```python
from build123d import *

# Parameters (mm, degrees)
BOSS_EXTRUDE1_DEPTH = 15
SKETCH3_R           = 5
CUT_EXTRUDE1_DEPTH  = 13
CUT_EXTRUDE2_START  = -7
SKETCH4_R           = 10.1
CUT_EXTRUDE2_DEPTH  = 2.6
SKETCH5_R           = 1.75
CUT_EXTRUDE3_DEPTH  = 131.953306572
CUT_EXTRUDE4_START  = -8
SKETCH6_R           = 3
CUT_EXTRUDE4_DEPTH  = 123.953306572
FILLET1_START       = -130
FILLET1_DEPTH       = 19.4
CUT_EXTRUDE5_DEPTH  = 8


with BuildPart() as part:
    # Sketch1 → Boss-Extrude1 (new body)
    with BuildSketch(Plane.XY):
        with BuildLine():
            Line((-124.6, 14.6), (-128.493415545, 7.856406461))
            ThreePointArc((-128.493415545, 7.856406461), (-128.793116813, 7.132863596), (-128.895339334, 6.356406461))
            Line((-128.895339334, 6.356406461), (-128.895339334, -9.356406461))
            ThreePointArc((-128.895339334, -9.356406461), (-128.793116813, -10.132863596), (-128.493415545, -10.856406461))
            Line((-128.493415545, -10.856406461), (-124.6, -17.6))
            Line((-124.6, -17.6), (-110.6, -17.6))
            Line((-110.6, -17.6), (-110.6, -5))
            Line((-110.6, -5), (-110.6, 5))
            Line((-110.6, 5), (-110.6, 13.771572875))
            ThreePointArc((-110.6, 13.771572875), (-110.752240935, 14.53693974), (-111.185786438, 15.185786438))
            Line((-111.185786438, 15.185786438), (-111.6, 15.6))
            Line((-111.6, 15.6), (-123.6, 15.6))
            Line((-123.6, 15.6), (-124.6, 14.6))
        make_face()
    extrude(amount=BOSS_EXTRUDE1_DEPTH)

    # Sketch3 → Cut-Extrude1 (cut)
    with BuildSketch(Plane(origin=(-110.6, 0, 0), x_dir=(0, 0, -1), z_dir=(1, 0, 0))):
        Circle(SKETCH3_R)
    extrude(amount=-CUT_EXTRUDE1_DEPTH, mode=Mode.SUBTRACT)

    # Sketch4 → Cut-Extrude2 (cut, symmetric)
    with BuildSketch(Plane(origin=(-110.6, 0, 0), x_dir=(0, 0, -1), z_dir=(1, 0, 0)).offset(CUT_EXTRUDE2_START)):
        Circle(SKETCH4_R)
    extrude(amount=CUT_EXTRUDE2_DEPTH, both=True, mode=Mode.SUBTRACT)

    # Sketch5 → Cut-Extrude3 (cut, through all)
    with BuildSketch(Plane(origin=(0, 0, 0), x_dir=(-1, 0, 0), z_dir=(0, 0, -1))):
        with Locations((117.6, 12.85)):
            Circle(SKETCH5_R)
        with Locations((117.6, -12.85)):
            Circle(SKETCH5_R)
    extrude(amount=-CUT_EXTRUDE3_DEPTH, mode=Mode.SUBTRACT)

    # Sketch6 → Cut-Extrude4 (cut, through all)
    with BuildSketch(Plane(origin=(0, 0, 0), x_dir=(-1, 0, 0), z_dir=(0, 0, -1)).offset(CUT_EXTRUDE4_START)):
        with Locations((117.6, 12.85)):
            Circle(SKETCH6_R)
        with Locations((117.6, -12.85)):
            Circle(SKETCH6_R)
    extrude(amount=-CUT_EXTRUDE4_DEPTH, mode=Mode.SUBTRACT)

    # Fillet1: read off the stored shape, not the designer's step
    # Fillet1 outline → Fillet1 (cut)
    with BuildSketch(Plane.YZ.offset(FILLET1_START)):
        with BuildLine():
            ThreePointArc((-17.6, 5), (-14.671067812, 12.071067812), (-7.6, 15))
            Line((-7.6, 15), (-17.6, 15))
            Line((-17.6, 15), (-17.6, 5))
        make_face()
        with BuildLine():
            ThreePointArc((5.6, 15), (12.671067812, 12.071067812), (15.6, 5))
            Line((15.6, 5), (15.6, 15))
            Line((15.6, 15), (5.6, 15))
        make_face()
    extrude(amount=FILLET1_DEPTH, mode=Mode.SUBTRACT)

    # Sketch7 → Cut-Extrude5 (cut)
    with BuildSketch(Plane(origin=(0, 0, 0), x_dir=(-1, 0, 0), z_dir=(0, 0, -1))):
        Polygon((115, -8.6), (124.2, -8.6), (126.2, -6.6), (126.2, 6.6), (124.2, 8.6), (115, 8.6), align=None)
    extrude(amount=-CUT_EXTRUDE5_DEPTH, mode=Mode.SUBTRACT)


solid = part.part
```
Source: CAD feature listing. Evaluate the final solid. Frame: model axes, mm. A direction names the side the tool comes from. Give positions to 0.01 mm unless a question says otherwise; leave off trailing zeros. Write each loop counter-clockwise with the first axis right and the second up, starting at its lowest first coordinate (ties: lowest second). Pieces come first, ordered by that corner, then holes. Notation, with made-up numbers: (61.5, 9) - (120.5, 9) arc R21 cw to (120.5, 29) - close; hole circle Ø2 at (61.5, 36). An arc over 180 degrees is marked (long way). One line per item, written item: value. Start each with the question number.
Q1. Draft query along Y for faces 1 (the face through (-126.574, -14.181, 5.52)), 2 (the face through (-120, -1, 15)), 3 (the face through (-115.85, 12.93, 3.94)). Return one class per face: +Y half, -Y half, draft (parallel to the pull), parting line (faces both ways), or undercut.
Q2. Set-up query: faces 4 (the face through (-125.2, 7.6, 3.9)), 5 (the face through (-115.85, -12.77, 3.94)), 6 (the face through (-119, 11, 8)), 7 (the face through (-113, 0, 5)), 8 (the face through (-128, -1, 0)). Return all of +Z, -Z, +X, -X, +Y, -Y with unobstructed straight access to the full face (end or side cutting, diameter ignored); none if empty.
Q3. Section query B-B, the plane y = 12.85. Return the cut outline in (x, z).
Q4. Section query D-D, the plane z = 2.25. Return the cut outline in (x, y), then the cut area to 3 significant figures.
Q5. Section query A-A, the plane x = -117. Count the separate pieces of the cut face and the enclosed holes in it, then the cut area to 3 significant figures.
Q6. First-contact query: pin 1 Ø3 at (x, y) = (-117.6, 12.85) entering from +Z; pin 2 Ø8 at (x, y) = (-117.6, -12.85) entering from -Z; pin 3 Ø5.5 at (x, y) = (-118.5, 2.5) entering from -Z; pin 4 Ø5 at (x, y) = (-118.5, -13) entering from +Z. Flat tips, straight axial feed; report the tip coordinate or a pass-through.
Q7. Section query C-C, the plane z = 7. Return the cut outline in (x, y).
Q8. Material intervals for probe 1 along Y at (x, z) = (-117.6, 6); probe 2 along Y at (x, z) = (-117.6, 3.5); probe 3 along X at (y, z) = (6, 2), sorted ascending. Write a range as from..to.
Answer:
1. face 1: -Y half
1. face 2: draft
1. face 3: undercut
2. face 4: -Z
2. face 5: +Z, -Z
2. face 6: +Z
2. face 7: -Z, +X
2. face 8: -Z, +X, -X, +Y, -Y
3. outline: (-125.61, 0) - (-119.35, 0) - (-119.35, 8) - (-120.6, 8) - (-120.6, 11.89) - (-125.61, 11.89) - close; (-115.85, 0) - (-110.6, 0) - (-110.6, 11.89) - (-114.6, 11.89) - (-114.6, 8) - (-115.85, 8) - close
4. outline: (-128.9, -9.36) arc R3 ccw to (-128.49, -10.86) - (-124.6, -17.6) - (-110.6, -17.6) - (-110.6, -4.47) - (-115, -4.47) - (-115, -9.85) - (-120.2, -9.85) - (-120.2, -8.6) - (-124.2, -8.6) - (-126.2, -6.6) - (-126.2, 6.6) - (-124.2, 8.6) - (-120.2, 8.6) - (-120.2, 9.85) - (-115, 9.85) - (-115, 4.47) - (-110.6, 4.47) - (-110.6, 13.77) arc R2 ccw to (-111.19, 15.19) - (-111.6, 15.6) - (-123.6, 15.6) - (-124.6, 14.6) - (-128.49, 7.86) arc R3 ccw to (-128.9, 6.36) - close; hole circle Ø3.5 at (-117.6, -12.85); hole circle Ø3.5 at (-117.6, 12.85)
4. area: 310 mm2
5. separate pieces: 3
5. enclosed holes: 0
5. area: 185 mm2
6. pin 1: passes through
6. pin 2: stops at z = 0
6. pin 3: stops at z = 8
6. pin 4: stops at z = 14.43
7. outline: (-128.9, -9.36) arc R3 ccw to (-128.49, -10.86) - (-124.72, -17.4) - (-110.6, -17.4) - (-110.6, 13.77) arc R2 ccw to (-111.19, 15.19) - (-111.4, 15.4) - (-123.8, 15.4) - (-124.6, 14.6) - (-128.49, 7.86) arc R3 ccw to (-128.9, 6.36) - close; hole (-126.2, -6.6) - (-124.2, -8.6) - (-115, -8.6) - (-115, 8.6) - (-124.2, 8.6) - (-126.2, 6.6) - close; hole circle Ø3.5 at (-117.6, -12.85); hole circle Ø3.5 at (-117.6, 12.85)
8. probe 1: y = -17.55..-14.6, -11.1..-8.6, 8.6..11.1, 14.6..15.55
8. probe 2: y = -17.6..-14.6, -11.1..-9.47, 9.47..11.1, 14.6..15.6
8. probe 3: x = -128.9..-126.2, -115..-110.6
